Autodesk Fusion 360 part; units mm, degrees
sketch "Sketch1" plane through (0, 0, 0) normal (0, 0, 1) x (1, 0, 0)
  line L0 (20, -10) -> (-20, -10)
  line L1 (-20, -10) -> (-20, 10)
  line L2 (-20, 10) -> (20, 10)
  line L3 (20, 10) -> (20, -10)
  line L4 (20, -10) -> (-20, 10) construction
  line L5 (-20, -10) -> (20, 10) construction
  line L6 (10, 10) -> (10, -10)
  line L7 (-10, 10) -> (-10, -10) construction
  circle A0 centre (-10, 0) radius 1.7
  circle A1 centre (-10, 0) radius 3
  circle A2 centre (10, 0) radius 1.45
  circle A3 centre (10, 0) radius 3
  line L8 (-20, 3) -> (20, 3)
  line L9 (-20, -3) -> (20, -3)
  circle A4 centre (10, 0) radius 6
  line L10 (13, 5.1962) -> (13, 10)
  line L11 (7, 5.1962) -> (7, 10)
  line L12 (-7, 3) -> (-7, -3)
  line L13 (7, 3) -> (7, -3)
  line L14 (0, 10) -> (0, -10)
  line L15 (-20, 10) -> (-40, 10)
  line L16 (-40, 10) -> (-40, -10)
  line L17 (-40, -10) -> (-20, -10)
  line L18 (-40, 0) -> (-20, 0) construction
  circle A5 centre (-30, 0) radius 1.7
  circle A6 centre (-30, 0) radius 3
  dimension "d1" = 40
  dimension "d2" = 20
  dimension "d3" = 10
  dimension "d4" = 10
  dimension "d5" = 3.4
  dimension "d6" = 6
  dimension "d7" = 12
  dimension "d8" = 6
  dimension "d15" = 2.9
  dimension "d36" = 20
extrude "Extrude1" add sketch "Sketch1" against normal blind 1.2 contours L8 L9 A4 L14 | L8 L9 L12 L14 | L8 L9 A4 L13
extrude "Extrude2" add sketch "Sketch1" along normal blind 39.5 contours L0 L3 L6 L9 A4 | L0 L6 L9 A4 L14 | L3 L8 L9 A4 | L6 L9 A4 | L6 L9 A4 | L2 L3 L8 A4 L10 | A3 L8 L9 A4 | L8 L9 A4 L14 | L6 A2 A3 | A3 L9 L13 | L6 A2 A3 | L8 L9 A4 L13 | L6 L8 A4 | L2 L8 A4 L11 L14 | L6 A2 | L6 A2 | A3 L8 L13 | L6 L8 A4 | L2 L6 A4 L10 | L2 L6 A4 L11
extrude "Extrude3" cut sketch "Sketch1" along normal blind 39.5 contours L6 A2 | L6 A2
extrude "Extrude4" add sketch "Sketch1" along normal blind 29.5 contours L6 A2 | L6 A2
extrude "Extrude5" add sketch "Sketch1" along normal blind 5 contours L0 L1 L9 L14 | L1 L15 L16 L17 | L8 L9 L12 L14 | L1 A1 L8 L9 | A1 L9 L12 | L1 L2 L8 L14 | A1 | A1 L8 L12 | A6
extrude "Extrude6" add sketch "Sketch1" along normal blind 3 from surface at 5 contours L0 L1 L9 L14 | L1 L15 L16 L17 | L8 L9 L12 L14 | L1 A1 L8 L9 | A1 L9 L12 | L1 L2 L8 L14 | A1 L8 L12
extrude "Extrude8" add sketch "Sketch1" along normal blind 10 from surface at 39.5 contours L0 L3 L6 L9 A4 | L0 L6 L9 A4 L14 | L3 L8 L9 A4 | L2 L3 L8 A4 L10 | L8 L9 A4 L14 | L2 L8 A4 L11 L14
fillet "Fillet3" radius 3 2 edges at (7, 5.1962, 44.5) (13, 5.1962, 44.5)
draft "Draft1" angle 8 neutral plane through (0, 0, 49.5) pull (0, 0, 1) 1 faces at (0, 3.3333, 21.8333)
fillet "Fillet1" radius 3 6 edges at (20, -10, 24.75) (20, 10, 24.75) (-2.9162, 10, 28.75) (-2.9162, -10, 28.75) (-40, -10, 4) (-40, 10, 4)
chamfer "Chamfer1" distance 0.4 angle 45 2 edges at (-12.797, 1.0848, 8) (-32.797, 1.0848, 8)
chamfer "Chamfer2" distance 0.2 angle 45 2 edges at (-11.585, 0.6147, 5) (-31.585, 0.6147, 5)
chamfer "Chamfer3" distance 0.2 angle 45 1 edges at (8.6481, 0.5243, 39.5)
chamfer "Chamfer4" distance 1 angle 45 5 edges at (-19.9015, 10, 8) (-39.1213, 9.1213, 8) (-40, 0, 8) (-39.1213, -9.1213, 8) (-19.9015, -10, 8)
extrude "Extrude7" cut 1 faces at (-2.3333, 1, -1.2) along direction (0, 0, 1) blind 1.2
chamfer "Chamfer5" distance 0.4 angle 45 1 faces at (8.5667, 0, 0)
fillet "Fillet4" radius 1.5 2 edges at (7, 10, 44.5) (13, 10, 44.5)
chamfer "Chamfer6" distance 1 angle 45 16 edges at (0, 0, 49.5) (0.8873, -9.1213, 49.5) (10.0147, -10, 49.5) (19.1213, -9.1213, 49.5) (20, 0, 49.5) (19.1213, 9.1213, 49.5) (15.75, 10, 49.5) (13.4393, 9.5607, 49.5) (13, 7.6041, 49.5) (13.2614, 5.4835, 49.5) (10, -6, 49.5) (6.7386, 5.4835, 49.5) (7, 7.6041, 49.5) (6.5607, 9.5607, 49.5) (4.2647, 10, 49.5) (0.8873, 9.1213, 49.5)
equation "d9 = -( 2 mm - 0.8 mm )"
equation "d16 = 39.50 mm - 10 mm"
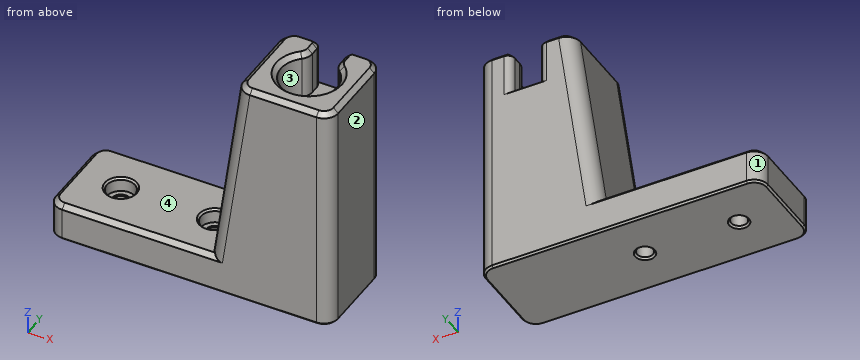
Geometry check sheet. Reference: the model listing, model coordinates, mm. Face numbers are marked on the shaded views. Round coordinates to 2 decimals unless told otherwise and drop trailing zeros. Loops run counter-clockwise (first coordinate to the right, second up) from the corner with the lowest first, then second, coordinate; pieces in that order, holes last. Notation, with made-up numbers: (35.25, 7) -> (85.25, 7) arc R26 ccw to (85.25, 31) -> close; hole circle Ø3 at (-9, 21). An arc over 180 degrees is marked (long way). Use a Markdown table: item, result.
(1) Sectioned sample at C-C (x = -25.5). Enter the section's corners in (y, z), then the cut area to 3 significant figures.
Calculated:
| item | result |
|---|---|
| outline | (-10, 0.4) -> (-9.6, 0) -> (9.6, 0) -> (10, 0.4) -> (10, 7) -> (9, 8) -> (-9, 8) -> (-10, 7) -> close |
| area | 159 mm² |
(2) Go/stop test with flat-tipped pins: P1, Ø3, axis at x = -31, y = 1, coming from the +Z side; P2, Ø3, axis at x = -10, y = 0, coming from the +Z side; P3, Ø12, axis at y = -1, z = 36, coming from the -X side; P4, Ø3, axis at y = 4, z = 35.5, coming from the -X side. Record where each tip stops, or that it passes through.
Calculated:
| item | result |
|---|---|
| P1 | z = 5 |
| P2 | through |
| P3 | x = -2.74 |
| P4 | x = -2.18 |
(3) Sectioned sample at D-D (x = 10). Enter the section's corners in (y, z).
Calculated:
| item | result |
|---|---|
| outline | (-10, 0.4) -> (-9.6, 0) -> (9.6, 0) -> (10, 0.4) -> (10, 39.5) -> (1.65, 39.5) -> (1.45, 39.3) -> (1.45, 29.5) -> (-1.45, 29.5) -> (-1.45, 39.3) -> (-1.65, 39.5) -> (-6, 39.5) -> (-6, 48.5) -> (-7, 49.5) -> (-9, 49.5) -> (-10, 48.5) -> close |
(4) Sectioned sample at A-A (x = -10). Enter the section's corners in (y, z), then the cut area to 3 significant figures.
Calculated:
| item | result |
|---|---|
| outline | (-10, 0.4) -> (-9.6, 0) -> (-2.1, 0) -> (-1.7, 0.4) -> (-1.7, 4.8) -> (-1.9, 5) -> (-3, 5) -> (-3, 7.6) -> (-3.4, 8) -> (-9, 8) -> (-10, 7) -> close; (1.7, 0.4) -> (2.1, 0) -> (9.6, 0) -> (10, 0.4) -> (10, 7) -> (9, 8) -> (3.4, 8) -> (3, 7.6) -> (3, 5) -> (1.9, 5) -> (1.7, 4.8) -> close |
| area | 123 mm² |
(5) Sectioned sample at B-B (y = 0). Give the number of separate pieces and of enclosed holes in the cut face, then the cut area to 3 significant figures.
Calculated:
| item | result |
|---|---|
| separate pieces | 3 |
| enclosed holes | 0 |
| area | 1,210 mm² |
(6) Scan lines: probe 1 along Y at (x, z) = (-10, 1.95); probe 2 along Y at (x, z) = (-30, 6.95); probe 3 along Z at (x, y) = (-33.5, 9). Record each from-to range of solid material in increasing order.
Calculated:
| item | result |
|---|---|
| probe 1 | -10 to -1.7, 1.7 to 10 |
| probe 2 | -10 to -3, 3 to 10 |
| probe 3 | 0 to 8 |
(7) Mould release check, pull along X, two halves, no side actions. Record for the marked faces 1, 2, 3 and 4: released by +X, released by -X, zero draft, split by the parting line, or undercut.
Calculated:
| item | result |
|---|---|
| face 1 | released by -X |
| face 2 | released by +X |
| face 3 | undercut |
| face 4 | zero draft |
